Could you check a few things on this drawing? It's one solid part, dimensions in mm from its lowest x, y, z. A direction names the side the tool comes from. Give positions to 0.01 mm unless a question says otherwise; leave off trailing zeros. Loops run counter-clockwise (first coordinate to the right, second up) from the corner with the lowest first, then second, coordinate; pieces in that order, holes last. Notation, with made-up numbers: (45, -8) - (50, -8) arc R28 cw to (50, 12) - close; hole circle Ø11 at (-34, 38). An arc over 180 degrees is marked (long way). Return JSON: item names as keys, results as strings. Group by question number.
(1) If we section it at C-C (x = 3): Please give me the cut outline in (y, z).
(2) I need wall thicknesses on probe 1 along Y at (x, z) = (12.5, 28); probe 2 along Y at (x, z) = (5.25, 28); probe 3 along Z at (x, y) = (4.5, 48.5). Which ranges of each line are inside material? Lowest first, please. Write a range as [from, to].
(3) If we section it at A-A (z = 28): Please give me the cut outline in (x, y), then the cut area to 3 significant figures.
(4) For P1, Ø5, axis at x = 12, y = 46.5, coming from the +Z side; P2, Ø2, axis at x = 3.5, z = 35.5, coming from the +Y side; P3, Ø1.5, axis at y = 17, z = 50, coming from the -X side; P4, Ø6, axis at x = 8, y = 25, coming from the -Z side, each with a flat end and sliding along its axis, tell me the tip position at first contact or that it passes through.
(5) On a 3-axis mill with a long thin cutter (end or side, diameter ignored), from which of +Z, -Z, +X, -X, +Y, -Y can I reach the whole of each face in a straight line? I mean the marked faces 3 and 4. Say none if no direction works.
(6) If we mould it in two halves opening along Y, with no side actions, what happens to the marked faces 1 and 2? For each: released by +Y, released by -Y, zero draft, split by the parting line, or undercut.
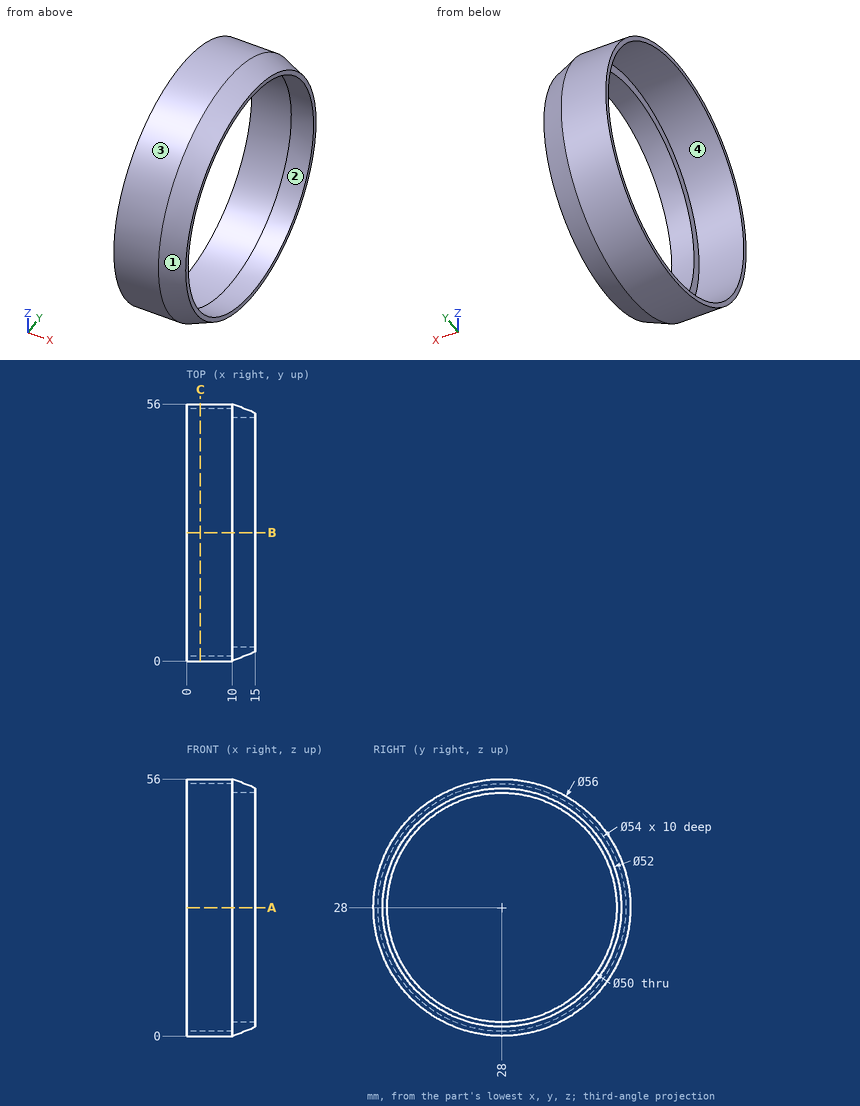
Values:
{
 "1": {"outline": "circle Ø56 at (28, 28); hole circle Ø54 at (28, 28)"},
 "2": {"probe 1": "[1, 3], [53, 55]", "probe 2": "[0, 1], [55, 56]", "probe 3": "[8.93, 10.43], [45.57, 47.07]"},
 "3": {"outline": "(0, 0) - (10, 0) - (15, 2) - (15, 3) - (10, 3) - (10, 1) - (0, 1) - close; (0, 55) - (10, 55) - (10, 53) - (15, 53) - (15, 54) - (10, 56) - (0, 56) - close", "area": "40.0 mm2"},
 "4": {"P1": "z = 50.38", "P2": "y = 55.24", "P3": "x = 10", "P4": "z = 0"},
 "5": {"face 3": "+X, -X", "face 4": "-X"},
 "6": {"face 1": "split by the parting line", "face 2": "undercut"}
}
